Geometry: final body of the model. Coordinates: model frame, mm. Face numbers are marked on the shaded views. A direction names the side the tool comes from. Give positions to 0.01 mm unless a question says otherwise; leave off trailing zeros. Write each loop counter-clockwise with the first axis right and the second up, starting at its lowest first coordinate (ties: lowest second). Pieces come first, ordered by that corner, then holes. Notation, with made-up numbers: (27.25, -1) -> (31.25, -1) arc R14 ccw to (31.25, 4) -> close; hole circle Ø4 at (-37, 56). An arc over 180 degrees is marked (long way). Answer in a Markdown table with one row per item. Add a question column.
from build123d import *

# Parameters (mm, degrees)
SKETCH1_R           = 1.6
SKETCH1_R_2         = 5
SKETCH1_W           = 42
SKETCH1_H           = 22
BOSS_EXTRUDE1_DEPTH = 10
BOSS_EXTRUDE2_DEPTH = 10
BOSS_EXTRUDE4_START = 44.5
SKETCH2_R           = 5
BOSS_EXTRUDE4_DEPTH = 5
BOSS_EXTRUDE3_START = -10
SKETCH1_5_W         = 10
SKETCH1_5_H         = 50
BOSS_EXTRUDE3_DEPTH = 54.5
SKETCH3_R           = 3.5
CUT_EXTRUDE1_DEPTH  = 10
SKETCH4_R           = 5
SKETCH4_R_2         = 2.7
BOSS_EXTRUDE5_DEPTH = 10
BOSS_EXTRUDE6_START = 44.5
SKETCH4_2_R         = 5
SKETCH4_2_R_2       = 2.7
BOSS_EXTRUDE6_DEPTH = 5


with BuildPart() as part:
    # Sketch1 → Boss-Extrude1 (new body)
    with BuildSketch(Plane(origin=(0, 0, 0), x_dir=(1, 0, 0), z_dir=(0, 1, 0))):
        with BuildLine():
            Line((4.949747468, 4.949747468), (3.964466094, 5.935028843))
            ThreePointArc((3.964466094, 5.935028843), (2.880602337, 7.557145587), (2.5, 9.470562748))
            Line((2.5, 9.470562748), (2.5, 33))
            Line((2.5, 33), (-52.5, 33))
            Line((-52.5, 33), (-52.5, -7))
            Line((-52.5, -7), (0, -7))
            ThreePointArc((0, -7), (6.467156728, -2.678784027), (4.949747468, 4.949747468))
        make_face()
        with Locations((-49.3, 25)):
            Circle(SKETCH1_R, mode=Mode.SUBTRACT)
        with Locations((-49.3, 15)):
            Circle(SKETCH1_R, mode=Mode.SUBTRACT)
        with Locations((-0.7, 15)):
            Circle(SKETCH1_R, mode=Mode.SUBTRACT)
        with Locations((-0.7, 25)):
            Circle(SKETCH1_R, mode=Mode.SUBTRACT)
        Circle(SKETCH1_R_2, mode=Mode.SUBTRACT)
        with Locations((-25, 20)):
            Rectangle(SKETCH1_W, SKETCH1_H, mode=Mode.SUBTRACT)
    extrude(amount=-BOSS_EXTRUDE1_DEPTH)

    # Sketch1<4> → Boss-Extrude2 (add)
    with BuildSketch(Plane(origin=(0, 0, 0), x_dir=(1, 0, 0), z_dir=(0, 1, 0))):
        Polygon((-72.5, -7), (-52.5, -7), (-52.5, 33), (-72.5, 43), align=None)
    extrude(amount=-BOSS_EXTRUDE2_DEPTH)



with BuildPart() as body_2:
    # Sketch2 → Boss-Extrude4 (new body)
    with BuildSketch(Plane(origin=(0, 0, 0), x_dir=(1, 0, 0), z_dir=(0, 1, 0)).offset(BOSS_EXTRUDE4_START)):
        with BuildLine():
            Line((-72.5, 43), (-52.5, 33))
            Line((-52.5, 33), (3.032382393, 6.309093201))
            ThreePointArc((3.032382393, 6.309093201), (6.825088, -1.555047844), (0, -7))
            Line((0, -7), (-52.5, -7))
            Line((-52.5, -7), (-82.5, -7))
            Line((-82.5, -7), (-82.5, 43))
            Line((-82.5, 43), (-72.5, 43))
        make_face()
        Circle(SKETCH2_R, mode=Mode.SUBTRACT)
    extrude(amount=BOSS_EXTRUDE4_DEPTH)


with BuildPart() as part_1:
    add(part.part)

    add(body_2.part)  # Boss-Extrude3 merges body 2
    # Sketch1<5> → Boss-Extrude3 (add)
    with BuildSketch(Plane(origin=(0, 0, 0), x_dir=(1, 0, 0), z_dir=(0, 1, 0)).offset(BOSS_EXTRUDE3_START)):
        with Locations((-77.5, 18)):
            Rectangle(SKETCH1_5_W, SKETCH1_5_H)
    extrude(amount=BOSS_EXTRUDE3_DEPTH)

    # Sketch3 → Cut-Extrude1 (cut)
    with BuildSketch(Plane.ZY.offset(82.5)):
        with Locations((-3, 34.75)):
            Circle(SKETCH3_R)
        with Locations((-3, 4.75)):
            Circle(SKETCH3_R)
        with Locations((-33, 4.75)):
            Circle(SKETCH3_R)
        with Locations((-33, 34.75)):
            Circle(SKETCH3_R)
    extrude(amount=-CUT_EXTRUDE1_DEPTH, mode=Mode.SUBTRACT)

    # Sketch4 → Boss-Extrude5 (add)
    with BuildSketch(Plane(origin=(0, 0, 0), x_dir=(1, 0, 0), z_dir=(0, 1, 0))):
        Circle(SKETCH4_R)
        Circle(SKETCH4_R_2, mode=Mode.SUBTRACT)
    extrude(amount=-BOSS_EXTRUDE5_DEPTH)

    # Sketch4<2> → Boss-Extrude6 (add)
    with BuildSketch(Plane(origin=(0, 0, 0), x_dir=(1, 0, 0), z_dir=(0, 1, 0)).offset(BOSS_EXTRUDE6_START)):
        Circle(SKETCH4_2_R)
        Circle(SKETCH4_2_R_2, mode=Mode.SUBTRACT)
    extrude(amount=BOSS_EXTRUDE6_DEPTH)


solid = part_1.part
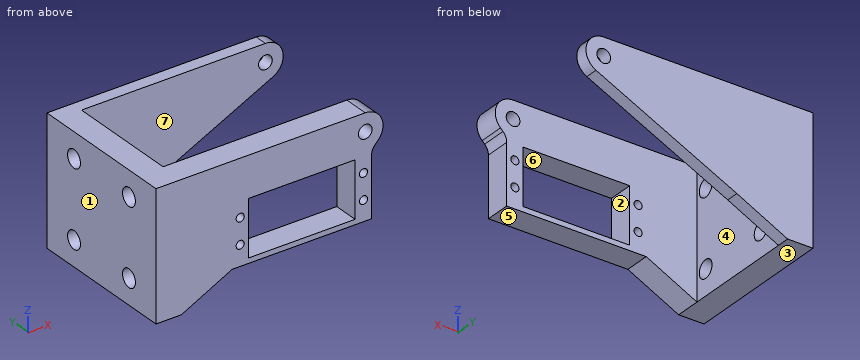
Q1. Line query: probe 1 along X at (y, z) = (-6, -15); probe 2 along Z at (x, y) = (-49.3, -4.75); probe 3 along Y at (x, z) = (-78.5, -3). Output: solid intervals per line, ascending. Write a range as from..to.
Q2. Section A-A on y = 4.75. Return loops of the section in (x, z), and give its area (3 significant figures).
Q3. Pull-direction query (X, two-part tool) for the marked faces 1, 2, 3 and 4; classes: +X half, -X half, draft (parallel to the pull), parting line (faces both ways), or undercut.
Q4. Section B-B on z = -21. Return loops of the section in (x, y).
Q5. Contact query for flat-ended pins moving along their axis: pin 1 Ø5 at (x, y) = (-25.5, -5.5) entering from -Z; pin 2 Ø8 at (y, z) = (34.75, -3) entering from +X; pin 3 Ø1.9 at (x, z) = (-49.3, -15) entering from -Y. Output: stop coordinate, or through.
Q6. Access query for the marked faces 5, 6 and 7. Directions: +Z, -Z, +X, -X, +Y, -Y. A direction counts if a zero-diameter tool reaches every point of the face in a straight line with its end or side. Return the directions, or none.
Q7. Section D-D on x = -49.3. Return loops of the section in (y, z).
Q8. Section C-C on z = -34. Return loops of the section in (x, y), and give its area (3 significant figures).
Checks:
| question | item | result |
|---|---|---|
| 1 | probe 1 | -82.5..-50.9, -47.7..-46, -4..-2.3, 0.9..2.5 |
| 1 | probe 2 | -33..-26.6, -23.4..-16.6, -13.4..7 |
| 1 | probe 3 | -10..1.25, 8.25..31.25, 38.25..49.5 |
| 2 | outline | (-82.5, -43) -> (-72.5, -43) -> (-72.5, -36.5) -> (-82.5, -36.5) -> close; (-82.5, -29.5) -> (-72.5, -29.5) -> (-72.5, -6.5) -> (-82.5, -6.5) -> close; (-82.5, 0.5) -> (-72.5, 0.5) -> (-72.5, 7) -> (-82.5, 7) -> close |
| 2 | area | 360 mm^2 |
| 3 | face 1 | -X half |
| 3 | face 2 | undercut |
| 3 | face 3 | draft |
| 3 | face 4 | +X half |
| 4 | outline | (-82.5, -10) -> (-46, -10) -> (-46, 0) -> (-72.5, 0) -> (-72.5, 44.5) -> (-27.53, 44.5) -> (-27.53, 49.5) -> (-82.5, 49.5) -> close; (-4, -10) -> (2.5, -10) -> (2.5, 0) -> (-4, 0) -> close |
| 5 | pin 1 | z = -33 |
| 5 | pin 2 | x = -72.5 |
| 5 | pin 3 | y = 44.5 |
| 6 | face 5 | -Z, +X, +Y, -Y |
| 6 | face 6 | -Y |
| 6 | face 7 | +Z, -Z, +X |
| 7 | outline | (-10, -33) -> (0, -33) -> (0, -26.6) -> (-10, -26.6) -> close; (-10, -23.4) -> (0, -23.4) -> (0, -16.6) -> (-10, -16.6) -> close; (-10, -13.4) -> (0, -13.4) -> (0, 7) -> (-10, 7) -> close; (44.5, -31.46) -> (49.5, -31.46) -> (49.5, 7) -> (44.5, 7) -> close |
| 8 | outline | (-82.5, -10) -> (-54.5, -10) -> (-54.5, 0) -> (-72.5, 0) -> (-72.5, 1.4) -> (-82.5, 1.4) -> close; (-82.5, 8.1) -> (-72.5, 8.1) -> (-72.5, 31.4) -> (-82.5, 31.4) -> close; (-82.5, 38.1) -> (-72.5, 38.1) -> (-72.5, 44.5) -> (-54.5, 44.5) -> (-54.5, 49.5) -> (-82.5, 49.5) -> close |
| 8 | area | 731 mm^2 |
